Answer from the drawing. Dimensions are ordinates in mm from the lowest x, y and z of the part. Round coordinates to 2 decimals unless told otherwise and drop trailing zeros. Write each loop counter-clockwise with the first axis right and the second up, starting at its lowest first coordinate (ties: lowest second). Pieces come first, ordered by that corner, then holes. Notation, with made-up numbers: (86.25, 27) - (90.25, 27) arc R30 cw to (90.25, 58) - close; hole circle Ø6 at (39, 61.5). An arc over 180 degrees is marked (long way). Write item = value, one per line. Start each with the question number.
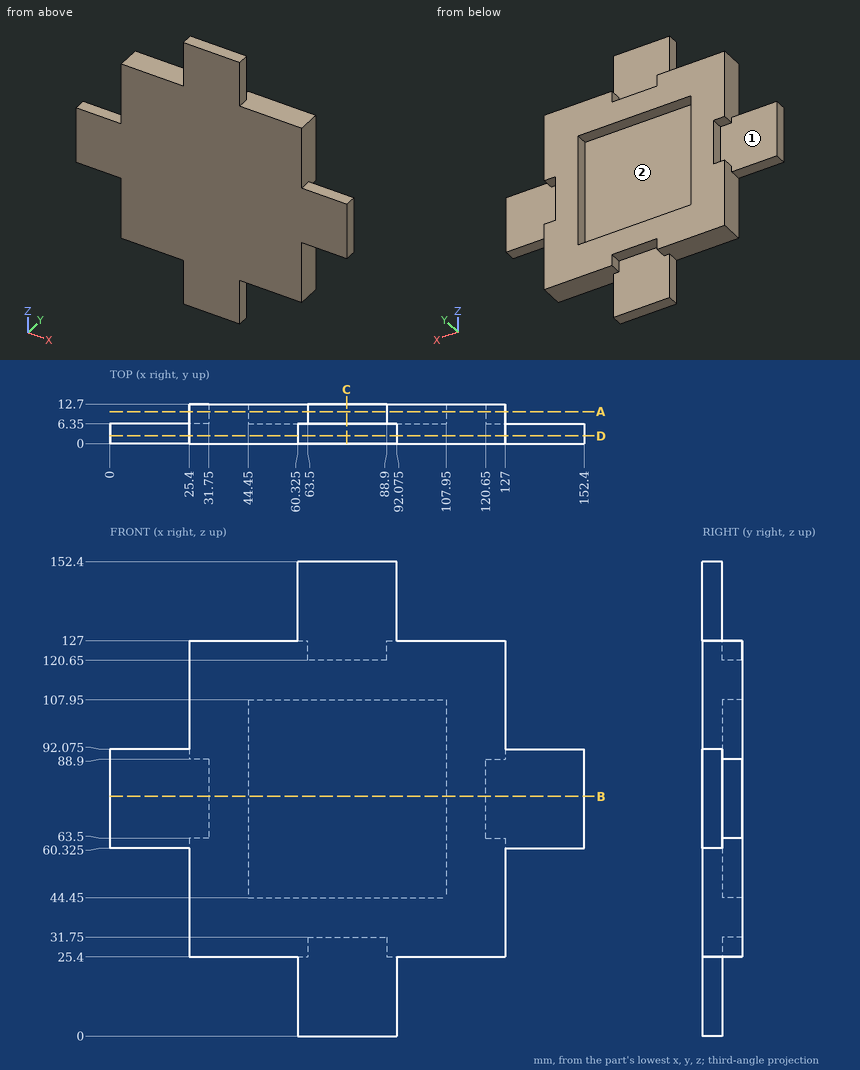
1. Consider line 1 (X direction, y = 7, z = 68); line 2 (Z direction, x = 123, y = 7.25); line 3 (Z direction, x = 54, y = 8.5). Determine where each line is inside the solid, lowest interval first.
2. Find section D-D on y = 2.5. Give the vertices of the cut face in (x, z) (3 decimals).
3. Find section A-A on y = 10.25. Give the vertices of the cut face in (x, z).
4. Each of these flat-tipped pins is pushed along its axis until it touches: pin 1 (7 mm diameter, centred on y = 8.5, z = 124, fed in from -X); pin 2 (3 mm diameter, centred on x = 131, y = 7, fed in from -Z) (3 decimals); pin 3 (4 mm diameter, centred on y = 10.5, z = 39, fed in from +X). Where does it stop, or does it pass through?
5. Find section B-B on z = 77. Give the vertices of the cut face in (x, y).
6. For a pull along X with two mould halves and no side action, classify the marked faces 1 and 2 as released by +X, released by -X, zero draft, split by the parting line, or undercut.
7. Find section C-C on x = 76. Give the vertices of the cut face in (y, z).
Answer key:
q1.line_1 = 31.75 to 44.45, 107.95 to 120.65
q1.line_2 = 25.4 to 63.5, 88.9 to 127
q1.line_3 = 25.4 to 44.45, 107.95 to 127
q2.outline = (0, 60.325) - (25.4, 60.325) - (25.4, 25.4) - (60.325, 25.4) - (60.325, 0) - (92.075, 0) - (92.075, 25.4) - (127, 25.4) - (127, 60.325) - (152.4, 60.325) - (152.4, 92.075) - (127, 92.075) - (127, 127) - (92.075, 127) - (92.075, 152.4) - (60.325, 152.4) - (60.325, 127) - (25.4, 127) - (25.4, 92.075) - (0, 92.075) - close
q3.outline = (25.4, 25.4) - (63.5, 25.4) - (63.5, 31.75) - (88.9, 31.75) - (88.9, 25.4) - (127, 25.4) - (127, 63.5) - (120.65, 63.5) - (120.65, 88.9) - (127, 88.9) - (127, 127) - (88.9, 127) - (88.9, 120.65) - (63.5, 120.65) - (63.5, 127) - (25.4, 127) - (25.4, 88.9) - (31.75, 88.9) - (31.75, 63.5) - (25.4, 63.5) - close; hole (44.45, 44.45) - (107.95, 44.45) - (107.95, 107.95) - (44.45, 107.95) - close
q4.pin_1 = 25.4
q4.pin_2 = 60.325
q4.pin_3 = 127
q5.outline = (0, 0) - (152.4, 0) - (152.4, 6.35) - (120.65, 6.35) - (120.65, 12.7) - (107.95, 12.7) - (107.95, 6.35) - (44.45, 6.35) - (44.45, 12.7) - (31.75, 12.7) - (31.75, 6.35) - (0, 6.35) - close
q6.face_1 = zero draft
q6.face_2 = undercut
q7.outline = (0, 0) - (6.35, 0) - (6.35, 31.75) - (12.7, 31.75) - (12.7, 44.45) - (6.35, 44.45) - (6.35, 107.95) - (12.7, 107.95) - (12.7, 120.65) - (6.35, 120.65) - (6.35, 152.4) - (0, 152.4) - close
